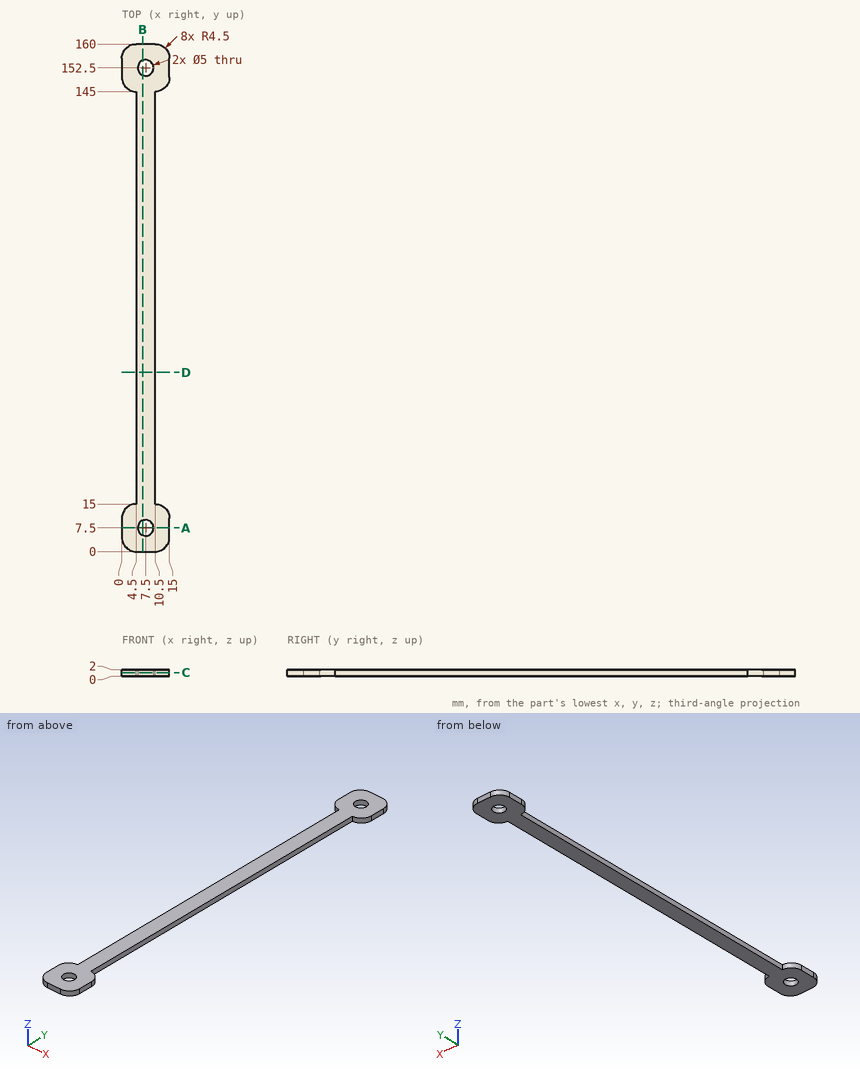
Check sheet for the drawn part. Datum: minimum x, y, z corner. Units: mm. Coordinates: 2 decimals unless noted, no trailing zeros. Write each loop counter-clockwise with the first axis right and the second up, starting at its lowest first coordinate (ties: lowest second). Pieces come first, ordered by that corner, then holes. Notation, with made-up numbers: M 76,74 L 110,74 A30 cw 110,100 Z; hole C -37,-4.75 d7. An arc over 180 degrees is marked long. One line per item, written item: value.
Item 1: Section check C-C, the plane z = 1.1. State how many separate pieces and enclosed holes the cut face has, plus the area to 3 significant figures.
Check sheet entries:
separate pieces: 1
enclosed holes: 2
area: 1,160 mm^2
Item 2: Scan lines: line 1 along Y through (x, z) = (7.5, 1.35); line 2 along X through (y, z) = (152.5, 1.6); line 3 along Y through (x, z) = (5.5, 1.1). Record each from-to range of solid material in increasing order.
Check sheet entries:
line 1: y = 0 to 5, 10 to 150, 155 to 160
line 2: x = 0 to 5, 10 to 15
line 3: y = 0 to 6, 9 to 151, 154 to 160
Item 3: Section check B-B, the plane x = 6.5. Record the boundary of the cut face in (y, z).
Check sheet entries:
outline: M 0,0 L 5.21,0 L 5.21,2 L 0,2 Z; M 9.79,0 L 150.21,0 L 150.21,2 L 9.79,2 Z; M 154.79,0 L 160,0 L 160,2 L 154.79,2 Z
Item 4: Section check A-A, the plane y = 7.5. Record the boundary of the cut face in (x, z), plus the area to 3 significant figures.
Check sheet entries:
outline: M 0,0 L 5,0 L 5,2 L 0,2 Z; M 10,0 L 15,0 L 15,2 L 10,2 Z
area: 20.0 mm^2
Item 5: Section check D-D, the plane y = 56.5. Record the boundary of the cut face in (x, z).
Check sheet entries:
outline: M 4.5,0 L 10.5,0 L 10.5,2 L 4.5,2 Z
Item 6: Gauge pin test, flat ends, axial feed: pin 1 Ø1 at (x, z) = (12, 0.5) entering from +Y; pin 2 Ø1 at (x, z) = (1.5, 0) entering from -Y. Record the tip position at first contact, or that the pin passes through.
Check sheet entries:
pin 1: stops at y = 159.89
pin 2: stops at y = 0.76
